Model file for the job. Use its own axes, mm. A direction names the side the tool comes from. Round coordinates to 2 decimals unless told otherwise and drop trailing zeros. Loops run counter-clockwise (first coordinate to the right, second up) from the corner with the lowest first, then second, coordinate; pieces in that order, holes last. Notation, with made-up numbers: (73.25, -38) -> (86.25, -38) arc R9 cw to (86.25, -31) -> close; hole circle Ø3 at (43, 82). An arc over 180 degrees is marked (long way). Use a Markdown table: item, result.
from build123d import *

# Parameters (mm, degrees)
F0_R     = 50
F1_DEPTH = 90
F2_R     = 41
F3_DEPTH = 50
F4_R     = 4
F5_DEPTH = 151
F6_R     = 41
F7_DEPTH = 3
F8_R     = 5.25
F9_DEPTH = 72


with BuildPart() as f1:
    # F0 (on Front) → F1 (new body)
    with BuildSketch(Plane.XZ):
        Circle(F0_R)
    extrude(amount=F1_DEPTH)

    # F2 (on face) → F3 (cut)
    with BuildSketch(Plane.XZ.offset(90)):
        Circle(F2_R)
    extrude(amount=-F3_DEPTH, mode=Mode.SUBTRACT)

    # F4 (on face) → F5 (cut)
    with BuildSketch(Plane(origin=(0, 0, 0), x_dir=(-1, 0, 0), z_dir=(0, 1, 0))):
        Circle(F4_R)
    extrude(amount=-F5_DEPTH, mode=Mode.SUBTRACT)

    # F6 (on face) → F7 (cut)
    with BuildSketch(Plane(origin=(0, 0, 0), x_dir=(-1, 0, 0), z_dir=(0, 1, 0))):
        Circle(F6_R)
    extrude(amount=-F7_DEPTH, mode=Mode.SUBTRACT)

    # F8 (on face) → F9 (cut)
    with BuildSketch(Plane.XZ.offset(40)):
        with Locations((0, 29)):
            Circle(F8_R)
        with Locations((0, -29)):
            Circle(F8_R)
    extrude(amount=-F9_DEPTH, mode=Mode.SUBTRACT)


solid = f1.part
Q1. Drill centre lines: L1, parallel to Z at x = 0, y = -32; L2, parallel to Z at x = 0, y = -68.5; L3, parallel to X at y = -51, z = -32. Where is each one in solid material? Low to high. Write a range as from..to.
Results list:
| item | result |
|---|---|
| L1 | z = -50..-34.25, -23.75..-4, 4..23.75, 34.25..50 |
| L2 | z = -50..-41, 41..50 |
| L3 | x = -38.42..-25.63, 25.63..38.42 |
Q2. Band-saw the part on D-D, the plane y = -43. Give the cut face in (x, z), plus the area to 3 significant figures.
Results list:
| item | result |
|---|---|
| outline | circle Ø100 at (0, 0); hole circle Ø82 at (0, 0) |
| area | 2,570 mm² |
Q3. Band-saw the part on B-B, the plane x = 0. Give the cut face in (y, z).
Results list:
| item | result |
|---|---|
| outline | (-90, -50) -> (0, -50) -> (0, -41) -> (-3, -41) -> (-3, -34.25) -> (-40, -34.25) -> (-40, -41) -> (-90, -41) -> close; (-90, 41) -> (-40, 41) -> (-40, 34.25) -> (-3, 34.25) -> (-3, 41) -> (0, 41) -> (0, 50) -> (-90, 50) -> close; (-40, -23.75) -> (-3, -23.75) -> (-3, -4) -> (-40, -4) -> close; (-40, 4) -> (-3, 4) -> (-3, 23.75) -> (-40, 23.75) -> close |
Q4. Flat gauge pins, fed straight in: pin 1 (24.5 mm diameter, centred on x = 8, z = 18, fed in from +Y); pin 2 (6 mm diameter, centred on x = -37.5, y = -65, fed in from -Z); pin 3 (8 mm diameter, centred on x = 31.5, y = -74.5, fed in from -Z). Where does each tip first touch, or does it go through?
Results list:
| item | result |
|---|---|
| pin 1 | stops at y = -3 |
| pin 2 | stops at z = -36.19 |
| pin 3 | stops at z = -41.76 |
Q5. Tool access for faces 1 (the face through (-9, -3, 1)), 2 (the face through (9, -40, 1)), 3 (the face through (2.42, -21.76, -33.66)): list every direction of +Z, -Z, +X, -X, +Y, -Y with a clear straight run to the whole face (end or side of a thin tool).
Results list:
| item | result |
|---|---|
| face 1 | +Y |
| face 2 | -Y |
| face 3 | +Y, -Y |
Q6. Band-saw the part on A-A, the plane z = 0. Give the cut face in (x, y), plus the area to 3 significant figures.
Results list:
| item | result |
|---|---|
| outline | (-50, -90) -> (-41, -90) -> (-41, -40) -> (-4, -40) -> (-4, -3) -> (-41, -3) -> (-41, 0) -> (-50, 0) -> close; (4, -40) -> (41, -40) -> (41, -90) -> (50, -90) -> (50, 0) -> (41, 0) -> (41, -3) -> (4, -3) -> close |
| area | 4,360 mm² |
Q7. Pull direction Z, two halves, no side cores. Call faces 4 (the face through (47.69, -44.37, 15.02)), 5 (the face through (-4, 0, 41)), 6 (the face through (9, -1, -40)): released by +Z, released by -Z, zero draft, split by the parting line, or undercut.
Results list:
| item | result |
|---|---|
| face 4 | split by the parting line |
| face 5 | zero draft |
| face 6 | undercut |
Q8. Band-saw the part on C-C, the plane z = 39. Give the cut face in (x, y), plus the area to 3 significant figures.
Results list:
| item | result |
|---|---|
| outline | (-31.29, -90) -> (-12.65, -90) -> (-12.65, -40) -> (12.65, -40) -> (12.65, -90) -> (31.29, -90) -> (31.29, 0) -> (12.65, 0) -> (12.65, -3) -> (-12.65, -3) -> (-12.65, 0) -> (-31.29, 0) -> close |
| area | 4,290 mm² |
